```python
from build123d import *

# Parameters (mm, degrees)
SZKIC1_R                    = 1.5
DODANIE_WYCI_GNI_CIE1_DEPTH = 10


with BuildPart() as part:
    # Szkic1 → Dodanie-wyciągnięcie1 (new body)
    with BuildSketch(Plane(origin=(0, 0, 0), x_dir=(1, 0, 0), z_dir=(0, 1, 0))):
        with BuildLine():
            Line((-15, -5), (17, -5))
            ThreePointArc((17, -5), (18.0250496, -4.929621344), (19.030861437, -4.719806218))
            add(Edge.make_bspline(
                [(21.050510257, -5), (20.034983278, -4.211064237), (19.030861437, -4.719806218)],
                knots=[0, 0, 0, 1, 1, 1], degree=2))
            ThreePointArc((21.050510257, -5), (24.855873501, -5.726702194), (27, -2.5))
            add(Edge.make_bspline(
                [(27, -2.5), (26, 2.5), (27, 7.5)],
                knots=[0, 0, 0, 1, 1, 1], degree=2))
            ThreePointArc((27, 7.5), (24.855873501, 10.726702194), (21.050510257, 10))
            add(Edge.make_bspline(
                [(21.050510257, 10), (20.034983278, 9.211064237), (19.030861437, 9.719806218)],
                knots=[0, 0, 0, 1, 1, 1], degree=2))
            ThreePointArc((19.030861437, 9.719806218), (18.0250496, 9.929621344), (17, 10))
            Line((17, 10), (-15, 10))
            ThreePointArc((-15, 10), (-16.314029759, 9.883991183), (-17.587409108, 9.539553545))
            add(Edge.make_bspline(
                [(-21.050510257, 10), (-19.428457916, 9.156413681), (-17.587409108, 9.539553545)],
                knots=[0, 0, 0, 1, 1, 1], degree=2))
            ThreePointArc((-21.050510257, 10), (-24.855873501, 10.726702194), (-27, 7.5))
            add(Edge.make_bspline(
                [(-27, 7.5), (-26, 2.5), (-27, -2.5)],
                knots=[0, 0, 0, 1, 1, 1], degree=2))
            ThreePointArc((-27, -2.5), (-24.855873501, -5.726702194), (-21.050510257, -5))
            add(Edge.make_bspline(
                [(-21.050510257, -5), (-19.486480964, -3.903838013), (-17.587409108, -4.539553545)],
                knots=[0, 0, 0, 1, 1, 1], degree=2))
            ThreePointArc((-17.587409108, -4.539553545), (-16.314029759, -4.883991183), (-15, -5))
        make_face()
        with Locations(Location((-23.5, -2.5, 0), (0, 0, 270))):
            Circle(SZKIC1_R, mode=Mode.SUBTRACT)
        with Locations(Location((-23.5, 7.5, 0), (0, 0, 270))):
            Circle(SZKIC1_R, mode=Mode.SUBTRACT)
        with Locations(Location((23.5, 7.5, 0), (0, 0, 270))):
            Circle(SZKIC1_R, mode=Mode.SUBTRACT)
        with Locations(Location((23.5, -2.5, 0), (0, 0, 270))):
            Circle(SZKIC1_R, mode=Mode.SUBTRACT)
        with BuildLine():
            Line((-15, 0), (15, 0))
            ThreePointArc((15, 0), (17.5, 2.5), (15, 5))
            Line((15, 5), (-15, 5))
            ThreePointArc((-15, 5), (-17.5, 2.5), (-15, 0))
        make_face(mode=Mode.SUBTRACT)
    extrude(amount=DODANIE_WYCI_GNI_CIE1_DEPTH)


solid = part.part
```
Geometry check sheet. Reference: the model listing, model coordinates, mm. A direction names the side the tool comes from. Give positions to 0.01 mm unless a question says otherwise; leave off trailing zeros. Write each loop counter-clockwise with the first axis right and the second up, starting at its lowest first coordinate (ties: lowest second). Pieces come first, ordered by that corner, then holes. Notation, with made-up numbers: (-37, -2.5) -> (22, -2.5) arc R19 cw to (22, 1.5) -> close; hole circle Ø11 at (23, -39.75). An arc over 180 degrees is marked (long way). One line per question, with ' | ' between items.
Item 1: Sectioned sample at C-C, the plane y = 3.5. State how many separate pieces and enclosed holes the cut face has, plus the area to 3 significant figures.
Determined:
separate pieces: 1 | enclosed holes: 5 | area: 610 mm^2
Item 2: Sectioned sample at A-A, the plane x = 23.5. Record the boundary of the cut face in (y, z).
Determined:
outline: (0, -11) -> (10, -11) -> (10, -9) -> (0, -9) -> close; (0, -6) -> (10, -6) -> (10, 1) -> (0, 1) -> close; (0, 4) -> (10, 4) -> (10, 6) -> (0, 6) -> close
Item 3: Access from +Z, -Z, +X, -X, +Y, -Y to the whole of each face (thin tool, end or side, straight path). Record for faces 3 (the flat face through (1, 5, -10)), 4 (the flat face through (0, 0, 1)), 5 (the flat face through (1, 5, 5)), 6 (the flat face through (0, 5, -5)).
Determined:
face 3: -Z, +Y, -Y | face 4: +Z, -Z, +X, -X, -Y | face 5: +Z, +Y, -Y | face 6: +Y, -Y
Item 4: Sectioned sample at B-B, the plane x = -1. Record the boundary of the cut face in (y, z), plus the area to 3 significant figures.
Determined:
outline: (0, -10) -> (10, -10) -> (10, -5) -> (0, -5) -> close; (0, 0) -> (10, 0) -> (10, 5) -> (0, 5) -> close | area: 100 mm^2
Item 5: Scan lines: line 1 along X through (y, z) = (7.75, -7.5); line 2 along Z through (x, y) = (6, 5); line 3 along Z through (x, y) = (24.5, 3.25). Record each from-to range of solid material in increasing order.
Determined:
line 1: -27 to -25, -22 to 22, 25 to 27 | line 2: -10 to -5, 0 to 5 | line 3: -10.85 to -8.62, -6.38 to 1.38, 3.62 to 5.85
Item 6: Sectioned sample at D-D, the plane x = -15.5. Record the boundary of the cut face in (y, z), plus the area to 3 significant figures.
Determined:
outline: (0, -9.98) -> (10, -9.98) -> (10, -4.95) -> (0, -4.95) -> close; (0, -0.05) -> (10, -0.05) -> (10, 4.98) -> (0, 4.98) -> close | area: 101 mm^2
Item 7: Depth check by flat-ended pin: pin 1 (5 mm diameter, centred on x = 23.5, z = 2.5, fed in from -Y); pin 2 (6 mm diameter, centred on y = 8, z = -3.5, fed in from +X); pin 3 (3 mm diameter, centred on x = -4.5, y = 5, fed in from +Z); pin 4 (3 mm diameter, centred on x = -12, y = 7.5, fed in from -Z). Enter the tip coordinate at first touch or a pass-through.
Determined:
pin 1: y = 0 | pin 2: x = 26.82 | pin 3: z = 5 | pin 4: z = -10
Item 8: Draft check along X on faces 1 (the flat face through (0, 10, 1)), 2 (the cylindrical face through (18.039, 4.93, -9.928)). Enter one of: released by +X, released by -X, zero draft, split by the parting line, or undercut.
Determined:
face 1: zero draft | face 2: undercut
